For this review, take the finished solid that the model builds, in its own axes (mm). Face numbers are marked on the shaded views. A direction names the side the tool comes from. Round coordinates to 2 decimals unless told otherwise and drop trailing zeros. Write each loop counter-clockwise with the first axis right and the second up, starting at its lowest first coordinate (ties: lowest second). Pieces come first, ordered by that corner, then holes. Notation, with made-up numbers: (-28, 64) -> (27, 64) arc R7 ccw to (27, 68) -> close; hole circle Ø11 at (-11.5, 35). An arc over 180 degrees is marked (long way). Write each question's results on one line, items separated by ' | '. Start each with the question number.
Item 1: Tool access review of the marked faces 4, 5 and 6: name each direction out of +Z, -Z, +X, -X, +Y, -Y from which nothing blocks a thin tool from reaching the whole face with its end or side.
Item 2: The part is to be moulded in two halves that separate along X. For the marked faces 1, 2 and 3, say which applies: +X half, -X half, draft (parallel to the pull), parting line (faces both ways), or undercut.
Item 3: Add section C-C (y = -8.5). State the section outline as (x, z) points, plus the area to 3 significant figures.
Item 4: Add section B-B (x = 10). State the section outline as (y, z) points.
Item 5: Add section A-A (z = 8.75). State the section outline as (x, y) points.
Item 6: Clearance check with flat-ended pins moving along their axes: pin 1 (3 mm diameter, centred on x = -12.5, z = 9, fed in from -Y); pin 2 (6 mm diameter, centred on x = 12, y = 2, fed in from +Z); pin 3 (7.5 mm diameter, centred on x = -7.5, z = 5.5, fed in from +Y). State where each tip first meets the part, or that it passes through.
Item 7: To check wall thickness, follow line 1 along Y through (x, z) = (-15.7, 1.25); line 2 along Y through (x, z) = (15.7, 0.55); line 3 along Y through (x, z) = (-3, 11.25). State the ranges of each line that lie inside material, in increasing order.
Item 8: Add section D-D (z = 5.5). State the section outline as (x, y) points.
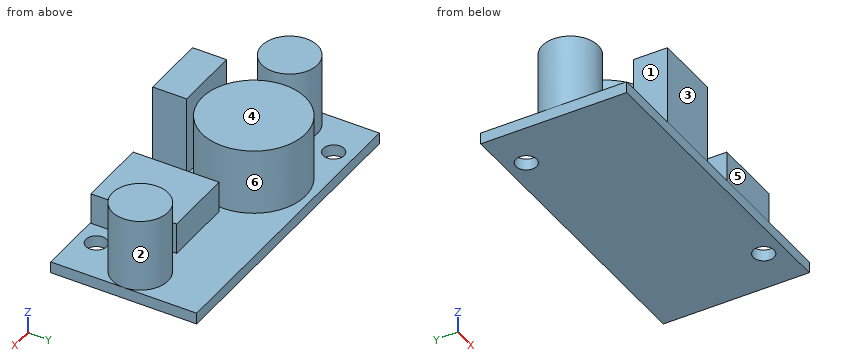
from build123d import *

# Parameters (mm, degrees)
SKETCH_1_W         = 44
SKETCH_1_H         = 21
SKETCH_1_R         = 1.5
EXTRUDE_484_DEPTH  = 1.65
SKETCH_2_R         = 4
EXTRUDE_1078_DEPTH = 10.5
SKETCH_2_3_W       = 9.6
SKETCH_2_3_H       = 4.9
EXTRUDE_1123_DEPTH = 11.5
SKETCH_2_4_R       = 7.45
EXTRUDE_1263_DEPTH = 9.5
SKETCH_2_5_W       = 10.2
SKETCH_2_5_H       = 12.35
EXTRUDE_1351_DEPTH = 4.5


with BuildPart() as part:
    # Sketch 1 → Extrude 484 (new body)
    with BuildSketch(Plane.XY):
        Rectangle(SKETCH_1_W, SKETCH_1_H)
        with Locations((-15.7, 7.7)):
            Circle(SKETCH_1_R, mode=Mode.SUBTRACT)
        with Locations((15.7, -7.7)):
            Circle(SKETCH_1_R, mode=Mode.SUBTRACT)
    extrude(amount=EXTRUDE_484_DEPTH)

    # Sketch 2 → Extrude 1078 (add)
    with BuildSketch(Plane.XY.offset(1.65)):
        with Locations(Location((-18, 0, 0), (0, 0, 180))):
            Circle(SKETCH_2_R)
        with Locations((18, 0)):
            Circle(SKETCH_2_R)
    extrude(amount=EXTRUDE_1078_DEPTH)

    # Sketch 2_3 → Extrude 1123 (add)
    with BuildSketch(Plane.XY.offset(1.65)):
        with Locations((-7.2, -7.95)):
            Rectangle(SKETCH_2_3_W, SKETCH_2_3_H)
    extrude(amount=EXTRUDE_1123_DEPTH)

    # Sketch 2_4 → Extrude 1263 (add)
    with BuildSketch(Plane.XY.offset(1.65)):
        with Locations((-6, 2)):
            Circle(SKETCH_2_4_R)
    extrude(amount=EXTRUDE_1263_DEPTH)

    # Sketch 2_5 → Extrude 1351 (add)
    with BuildSketch(Plane.XY.offset(1.65)):
        with Locations((7.4, -4.225)):
            Rectangle(SKETCH_2_5_W, SKETCH_2_5_H)
    extrude(amount=EXTRUDE_1351_DEPTH)


solid = part.part
Responses:
1) face 4: +Z, +Y | face 5: +Z, +X, -X, -Y | face 6: +Z
2) face 1: -X half | face 2: undercut | face 3: draft
3) outline: (-22, 0) -> (14.43, 0) -> (14.43, 1.65) -> (12.5, 1.65) -> (12.5, 6.15) -> (2.3, 6.15) -> (2.3, 1.65) -> (-2.4, 1.65) -> (-2.4, 13.15) -> (-12, 13.15) -> (-12, 1.65) -> (-22, 1.65) -> close; (16.97, 0) -> (22, 0) -> (22, 1.65) -> (16.97, 1.65) -> close | area: 225 mm^2
4) outline: (-10.5, 0) -> (10.5, 0) -> (10.5, 1.65) -> (1.95, 1.65) -> (1.95, 6.15) -> (-10.4, 6.15) -> (-10.4, 1.65) -> (-10.5, 1.65) -> close
5) outline: circle Ø8 at (-18, 0); circle Ø14.9 at (-6, 2); (-12, -10.4) -> (-2.4, -10.4) -> (-2.4, -5.5) -> (-12, -5.5) -> close; circle Ø8 at (18, 0)
6) pin 1: stops at y = -10.4 | pin 2: stops at z = 12.15 | pin 3: stops at y = 9.45
7) line 1: y = -10.5 to 6.2, 9.2 to 10.5 | line 2: y = -10.5 to -9.2, -6.2 to 10.5 | line 3: y = -10.4 to -5.5
8) outline: circle Ø8 at (-18, 0); circle Ø14.9 at (-6, 2); (-12, -10.4) -> (-2.4, -10.4) -> (-2.4, -5.5) -> (-12, -5.5) -> close; (2.3, -10.4) -> (12.5, -10.4) -> (12.5, 1.95) -> (2.3, 1.95) -> close; circle Ø8 at (18, 0)
